The model under review builds one solid part; all positions refer to its coordinate system, in mm. A direction names the side the tool comes from. Coordinates: 2 decimals unless noted, no trailing zeros. Order: outer loops, then holes, each group sorted by start corner. A loop starts at its lowest first (then second) coordinate and runs counter-clockwise, first axis right, second up. Notation, with made-up numbers: M 83.5,62 L 133.5,62 A32 ccw 133.5,89 Z; hole C -17,10 d7. An arc over 180 degrees is marked long. Answer in a Markdown table with one row per item.
from build123d import *

# Parameters (mm, degrees)
SKETCH1_W             = 28
SKETCH1_H             = 1
BOSS_EXTRUDE1_DEPTH   = 5
BOSS_EXTRUDE1_2_DEPTH = 5
BOSS_EXTRUDE2_DEPTH   = 1
BOSS_EXTRUDE3_DEPTH   = 11


with BuildPart() as part:
    # Sketch1 → Boss-Extrude1 (new body)
    with BuildSketch(Plane.XY):
        with Locations((14, 0.5)):
            Rectangle(SKETCH1_W, SKETCH1_H)
    extrude(amount=BOSS_EXTRUDE1_DEPTH)



with BuildPart() as body_2:
    # Sketch1 → Boss-Extrude1 2 (new body)
    with BuildSketch(Plane.XY):
        with Locations((14, 2.5)):
            Rectangle(SKETCH1_W, SKETCH1_H)
    extrude(amount=BOSS_EXTRUDE1_2_DEPTH)


with BuildPart() as part_1:
    add(part.part)

    add(body_2.part)  # Boss-Extrude2 merges body 2
    # Sketch2 → Boss-Extrude2 (add)
    with BuildSketch(Plane.XY.offset(5)):
        Polygon((0, 3), (28, 3), (28, 2), (23, 2), (23, 1), (28, 1), (28, 0), (0, 0), align=None)
    extrude(amount=BOSS_EXTRUDE2_DEPTH)

    # Sketch3 → Boss-Extrude3 (add)
    with BuildSketch(Plane.XY.offset(6)):
        Polygon((28, 3), (22, 3), (22, 0), (28, 0), (28, 1), (23, 1), (23, 2), (28, 2), align=None)
    extrude(amount=BOSS_EXTRUDE3_DEPTH)


solid = part_1.part
(1) Take a section at B-B (x = 26.5). Write out the cut boundary in (y, z).
Report:
| item | result |
|---|---|
| outline | M 0,0 L 1,0 L 1,17 L 0,17 Z; M 2,0 L 3,0 L 3,17 L 2,17 Z |
(2) Insertion check: P1, Ø1.5, axis at y = 0.5, z = 8, coming from the -X side; P2, Ø1, axis at x = 20, z = 13.5, coming from the -Y side; P3, Ø0.5, axis at y = 1.5, z = 13, coming from the +X side. Each pin has a flat end and moves straight along its axis. Give the tip position at first contact, or say it passes through.
Report:
| item | result |
|---|---|
| P1 | x = 22 |
| P2 | through |
| P3 | x = 23 |
(3) Take a section at C-C (y = 0.35). Write out the cut boundary in (x, z), then the cut area to 3 significant figures.
Report:
| item | result |
|---|---|
| outline | M 0,0 L 28,0 L 28,17 L 22,17 L 22,6 L 0,6 Z |
| area | 234 mm^2 |
(4) The part is to be moulded in two halves that separate along Y. For faces 4 (the flat face through (13.8, 2.5, 0)), 5 (the flat face through (17.3, 1, 4.6)), 6 (the flat face through (17, 3, 5)), say which applies: +Y half, -Y half, draft (parallel to the pull), parting line (faces both ways), or undercut.
Report:
| item | result |
|---|---|
| face 4 | draft |
| face 5 | undercut |
| face 6 | +Y half |
(5) Machinability: for faces 1 (the flat face through (11.7, 1.5, 5)), 2 (the flat face through (23, 1.5, 10.9)), 3 (the flat face through (16.9, 2, 4.6)), which of the approach directions +Z, -Z, +X, -X, +Y, -Y give a long, thin tool a straight path to every point of the face, cutting with its end or side? Answer none if there is none.
Report:
| item | result |
|---|---|
| face 1 | -Z, +X, -X |
| face 2 | +Z, -Z, +X |
| face 3 | -Z, +X |
(6) To check wall thickness, follow line 1 (Y direction, x = 5.5, z = 3.5); line 2 (X direction, y = 0.3, z = 8); line 3 (X direction, y = 1.6, z = 9.5). State the ranges of each line that lie inside material, in increasing order. Write a range as [from, to].
Report:
| item | result |
|---|---|
| line 1 | [0, 1], [2, 3] |
| line 2 | [22, 28] |
| line 3 | [22, 23] |
(7) Take a section at D-D (z = 6.5). Write out the cut boundary in (x, y), then the cut area to 3 significant figures.
Report:
| item | result |
|---|---|
| outline | M 22,0 L 28,0 L 28,1 L 23,1 L 23,2 L 28,2 L 28,3 L 22,3 Z |
| area | 13.0 mm^2 |
(8) Take a section at A-A (z = 3.25). Write out the cut boundary in (x, y), then the cut area to 3 significant figures.
Report:
| item | result |
|---|---|
| outline | M 0,0 L 28,0 L 28,1 L 0,1 Z; M 0,2 L 28,2 L 28,3 L 0,3 Z |
| area | 56.0 mm^2 |
